Autodesk Inventor part; units mm, degrees
ref_plane "YZ Plane" through (0, 0, 0) normal (1, 0, 0) x (0, 1, 0)
ref_plane "XZ Plane" through (0, 0, 0) normal (0, 1, 0) x (-1, 0, 0)
ref_plane "XY Plane" through (0, 0, 0) normal (0, 0, 1) x (1, 0, 0)
sketch "Boceto2" plane through (0, 0, 0) normal (0, 1, 0) x (-1, 0, 0)
  arc A0 (-18, 72.808) -> (20, 72.2842) centre (0, 0) ccw
  line L0 (-18, 72.808) -> (-18, 72.2842)
  line L1 (20, 72.2842) -> (13, 72.2842)
  line L2 (-18, 72.808) -> (-11, 72.808)
  line L3 (-11, 72.808) -> (-11, 72.2842)
  line L4 (-18, 72.2842) -> (-18, 72.808)
  line L5 (20, 72.2842) -> (13, 72.2842)
  line L6 (13, 72.2842) -> (20, 72.2842)
  line L7 (64.5832, 27.0002) -> (13, 27.0002)
  line L8 (13, 27.0002) -> (13, 72.2842)
  line L9 (-11, 72.2842) -> (-20, 72.2842)
  line L10 (-64.5832, 27.0002) -> (-11, 27.0002)
  line L11 (-11, 27.0002) -> (-11, 72.2842)
  arc A1 (69.8214, 4.9968) -> (69.8214, -4.9968) centre (70, 0) ccw
  arc A2 (-69.8214, -4.9968) -> (-69.8214, 4.9968) centre (-70, 0) ccw
  arc A3 (4.9968, -69.8214) -> (-4.9968, -69.8214) centre (0, -70) ccw
  arc A4 (4.9968, -69.8214) -> (69.8214, -4.9968) centre (0, 0) ccw
  arc A5 (69.8214, 4.9968) -> (64.5832, 27.0002) centre (0, 0) ccw
  arc A6 (-64.5832, 27.0002) -> (-69.8214, 4.9968) centre (0, 0) ccw
  arc A7 (-69.8214, -4.9968) -> (-4.9968, -69.8214) centre (0, 0) ccw
  dimension "d14" = 150
  dimension "d45" = 10
  dimension "d46" = 10
  dimension "d47" = 10
extrude "Extrusión2" add sketch "Boceto2" against normal blind 32 contours L9 L11 L10 A6 A2 A7 A3 A4 A1 A5 L7 L8 L1 A0
sketch "Boceto8" plane through (0, 0, 0) normal (0, 1, 0) x (-1, 0, 0)
  line L0 (59.5508, 67.2842) -> (-59.748, 67.2842)
  line L1 (-59.748, 67.2842) -> (-59.748, 82.2842)
  line L2 (-59.748, 82.2842) -> (59.5508, 82.2842)
  line L3 (59.5508, 82.2842) -> (59.5508, 67.2842)
  line L4 (13, 72.2842) -> (20, 72.2842)
  point P0 (0, 0)
  dimension "d67" = 15
  dimension "d71" = 5
extrude "Extrusión8" cut sketch "Boceto8" along normal mid plane 70
sketch "Boceto9" plane through (0, 0, 0) normal (0, 1, 0) x (-1, 0, 0)
  line L0 (-64.5832, 27.0002) -> (-11, 27.0002)
  line L1 (-23, 27.0002) -> (-64.5832, 27.0002)
  line L2 (-40.2309, 57.2842) -> (-23, 57.2842)
  line L3 (-23, 57.2842) -> (-23, 27.0002)
  line L4 (-11, 67.2842) -> (-11, 27.0002)
  line L5 (-33.1337, 67.2842) -> (-11, 67.2842)
  line L6 (25, 27.0002) -> (64.5832, 27.0002)
  line L7 (40.2309, 57.2842) -> (25, 57.2842)
  line L8 (25, 57.2842) -> (25, 27.0002)
  line L9 (13, 27.0002) -> (13, 67.2842)
  line L10 (13, 67.2842) -> (33.1337, 67.2842)
  arc A0 (-40.2309, 57.2842) -> (-64.5832, 27.0002) centre (0, 0) ccw
  arc A1 (64.5832, 27.0002) -> (40.2309, 57.2842) centre (0, 0) ccw
  dimension "d73" = 12
  dimension "d76" = 10
  dimension "d77" = 12
  dimension "d78" = 10
extrude "Extrusión9" cut sketch "Boceto9" against normal blind 32
sketch "Boceto15" plane through (0, 0, 0) normal (0, 1, 0) x (-1, 0, 0)
  circle A0 centre (0, 0) radius 73
  dimension "d126" = 146
extrude "Extrusión15" cut sketch "Boceto15" against normal blind 32
properties part number "Cuerpo" material "Aluminio 6061"
For this review, take the finished solid that the model builds, in its own axes (mm). Round coordinates to 2 decimals unless told otherwise and drop trailing zeros. Write each loop counter-clockwise with the first axis right and the second up, starting at its lowest first coordinate (ties: lowest second). Pieces come first, ordered by that corner, then holes. Notation, with made-up numbers: M 47,-17.75 L 101,-17.75 A12 ccw 101,-3.75 Z; hole C 13,-0.75 d3. An arc over 180 degrees is marked long. Write item = value, one per line. Start each with the question number.
(1) For line 1 along X through (y, z) = (-9.5, 0); line 2 along Z through (x, y) = (0, -19); line 3 along X through (y, z) = (-11, 47.5), list the stretches that pass through material, from the lowest coordinate up.
(2) We need section D-D (x = 0). Give the boundary of the cut face in (y, z), then the cut area to 3 significant figures.
(3) Clearance check with flat-ended pins moving along their axes: pin 1 Ø6 at (x, y) = (-23.5, -13.5) entering from -Z; pin 2 Ø8 at (x, y) = (56.5, -6.5) entering from +Z; pin 3 Ø1 at (y, z) = (-28, 41) entering from +X; pin 4 Ø10 at (x, z) = (-53, -35) entering from +Y. State where each tip first meets the part, or that it passes through.
(4) We need section A-A (z = 0). Give the boundary of the cut face in (x, y).
(5) We need section B-B (x = -57). Give the boundary of the cut face in (y, z), then the cut area to 3 significant figures.
(6) We need section C-C (y = -19). Give the boundary of the cut face in (x, z), then the cut area to 3 significant figures.
Results found:
q1.line_1 = -75 to -73, 73 to 75
q1.line_2 = -75 to -73
q1.line_3 = -58.04 to -55.43, 55.43 to 58.04
q2.outline = M -32,-75 L 0,-75 L 0,-73 L -32,-73 Z
q2.area = 64.0 mm²
q3.pin_1 = -72.14
q3.pin_2 = 53.56
q3.pin_3 = 63.12
q3.pin_4 = through
q4.outline = M -75,-32 L -73,-32 L -73,0 L -75,0 Z; M 73,-32 L 75,-32 L 75,0 L 73,0 Z
q5.outline = M -32,-48.74 L 0,-48.74 L 0,-45.61 L -32,-45.61 Z; M -32,45.61 L 0,45.61 L 0,48.74 L -32,48.74 Z
q5.area = 201 mm²
q6.outline = M -33.13,67.28 A75 ccw long 33.13,67.28 L 28.32,67.28 A73 cw long -28.32,67.28 Z
q6.area = 803 mm²
